Design review of the part built by this model. Coordinates are the model's own, in mm. A direction names the side the tool comes from. Coordinates: 2 decimals unless noted, no trailing zeros. Loops run counter-clockwise (first coordinate to the right, second up) from the corner with the lowest first, then second, coordinate; pieces in that order, holes last. Notation, with made-up numbers: (61, 42) -> (85, 42) arc R22 cw to (85, 77) -> close; hole circle Ø5 at (0.5, 54.5). An arc over 180 degrees is marked (long way). One line per item, written item: value. Start each with the question number.
1. Draft analysis for pull direction Z (two halves, no side actions). For faces 3 (the flat face through (-124.73, 0.021, -125.484)), 4 (the flat face through (-2, -1.511, -100)), 5 (the cylindrical face through (40.408, 0.021, -94.225)), 6 (the flat face through (-111.47, 0.02, -57.59)), state which applies: pulls with the +Z half, pulls with the -Z half, needs draft (parallel to the pull), parting line crosses it, or undercut.
2. Add section B-B on z = -55. Write out the cut boundary in (x, y), plus the area to 3 significant figures.
3. Machinability: for faces 1 (the flat face through (-64.801, 0.021, -20.804)), 2 (the flat face through (125.484, 0.021, -124.73)), which of the approach directions +Z, -Z, +X, -X, +Y, -Y give a long, thin tool a straight path to every point of the face, cutting with its end or side? Answer none if there is none.
4. For probe 1 along X at (y, z) = (0, -23); probe 2 along X at (y, z) = (-0.1, -66.5); probe 3 along Z at (x, y) = (71, -0.55), list the stretches that pass through material, from the lowest coordinate up.
5. Add section A-A on z = -81. Write out the cut boundary in (x, y).
6. Insertion check: pin 1 (1.5 mm diameter, centred on y = 0, z = -129, fed in from +X); pin 2 (3 mm diameter, centred on x = 24.46, z = -65.43, fed in from -Y); pin 3 (1 mm diameter, centred on x = 21, y = 0, fed in from +Z); pin 4 (1 mm diameter, centred on y = 1, z = -63, fed in from +X). Each pin has a flat end and moves straight along its axis. Give the tip position at first contact, or say it passes through.
7. Add section D-D on z = -142.5. Write out the cut boundary in (x, y) (3 decimals), plus the area to 3 significant figures.
8. Add section C-C on y = 1. Give the number of separate pieces and of enclosed holes in the cut face, plus the area to 3 significant figures.
```python
from build123d import *

# Parameters (mm, degrees)
BOSS_EXTRUDE1_DEPTH = 1.5113
SKETCH4_R           = 2.5527
CUT_EXTRUDE1_DEPTH  = 4.0226
CUT_EXTRUDE4_DEPTH  = 4.0226
SKETCH7_R           = 2.5527
CUT_EXTRUDE2_DEPTH  = 4.0226
SKETCH8_R           = 25.4
CUT_EXTRUDE3_DEPTH  = 4.0226


with BuildPart() as part:
    # Sketch3 → Boss-Extrude1 (new body, symmetric)
    with BuildSketch(Plane(origin=(0, 0, 0), x_dir=(1, 0, 0), z_dir=(0, 1, 0))):
        with BuildLine():
            Line((64.255461557, 10.37392483), (152.047852166, 98.16631544))
            Line((152.047852166, 98.16631544), (98.16631544, 152.047852166))
            Line((98.16631544, 152.047852166), (53.975, 152.047852166))
            Line((53.975, 152.047852166), (53.975, 120.65))
            Line((53.975, 120.65), (-53.975, 120.65))
            Line((-53.975, 120.65), (-53.975, 152.047852166))
            Line((-53.975, 152.047852166), (-98.16631544, 152.047852166))
            Line((-98.16631544, 152.047852166), (-152.047852166, 98.16631544))
            Line((-152.047852166, 98.16631544), (-64.255461557, 10.37392483))
            ThreePointArc((-64.255461557, 10.37392483), (0, 65.0875), (64.255461557, 10.37392483))
        make_face()
    extrude(amount=BOSS_EXTRUDE1_DEPTH, both=True)

    # Sketch4 → Cut-Extrude1 (cut, through all)
    with BuildSketch(Plane(origin=(0, 1.5113, 0), x_dir=(1, 0, 0), z_dir=(0, 1, 0))):
        with Locations((24.461985581, 65.426552419)):
            Circle(SKETCH4_R)
        with Locations((60.491874454, 34.925)):
            Circle(SKETCH4_R)
        with Locations((-60.491874454, 34.925)):
            Circle(SKETCH4_R)
        with Locations((-24.461985581, 65.426552419)):
            Circle(SKETCH4_R)
    extrude(amount=-CUT_EXTRUDE1_DEPTH, mode=Mode.SUBTRACT)

    # Sketch6 → Cut-Extrude4 (cut, through all)
    with BuildSketch(Plane(origin=(0, 1.5113, 0), x_dir=(1, 0, 0), z_dir=(0, 1, 0))):
        Polygon((69.743195158, 15.861658432), (60.762939037, 24.841914553), (59.718206073, 25.886647517), (64.255461557, 10.37392483), align=None)
    cut_extrude4 = extrude(amount=-CUT_EXTRUDE4_DEPTH, mode=Mode.SUBTRACT)

    # Sketch7 → Cut-Extrude2 (cut, through all)
    with BuildSketch(Plane(origin=(0, 1.5113, 0), x_dir=(1, 0, 0), z_dir=(0, 1, 0))):
        with Locations((70.865727173, 23.719382538)):
            Circle(SKETCH7_R)
        with Locations((79.845983295, 32.699638659)):
            Circle(SKETCH7_R)
    cut_extrude2 = extrude(amount=-CUT_EXTRUDE2_DEPTH, mode=Mode.SUBTRACT)

    # Mirror1: Cut-Extrude4, Cut-Extrude2 across plane
    add(cut_extrude4.mirror(Plane(origin=(0, 0, 0), x_dir=(0, 0, 1), z_dir=(1, 0, 0))), mode=Mode.SUBTRACT)
    add(cut_extrude2.mirror(Plane(origin=(0, 0, 0), x_dir=(0, 0, 1), z_dir=(1, 0, 0))), mode=Mode.SUBTRACT)

    # Sketch8 → Cut-Extrude3 (cut, through all)
    with BuildSketch(Plane(origin=(0, 1.5113, 0), x_dir=(1, 0, 0), z_dir=(0, 1, 0))):
        with Locations((59.128754095, 77.058092601)):
            Circle(SKETCH8_R)
    extrude(amount=-CUT_EXTRUDE3_DEPTH, mode=Mode.SUBTRACT)


solid = part.part
```
Worked answers:
1. face 3: pulls with the -Z half
1. face 4: needs draft
1. face 5: undercut
1. face 6: pulls with the +Z half
2. outline: (-108.88, -1.51) -> (-34.8, -1.51) -> (-34.8, 1.51) -> (-108.88, 1.51) -> close; (34.8, -1.51) -> (46.54, -1.51) -> (46.54, 1.51) -> (34.8, 1.51) -> close; (71.72, -1.51) -> (108.88, -1.51) -> (108.88, 1.51) -> (71.72, 1.51) -> close
2. area: 372 mm²
3. face 1: +Z, +Y, -Y
3. face 2: -Z, +X, +Y, -Y
4. probe 1: x = -76.88 to -73.31, -68.42 to -62.6, 62.6 to 68.42, 73.31 to 76.88
4. probe 2: x = -120.38 to -26.78, -22.15 to 22.15, 26.78 to 36.03, 82.23 to 120.38
4. probe 3: z = -152.05 to -99.51, -54.6 to -26.27, -21.17 to -17.12
5. outline: (-134.88, -1.51) -> (34.04, -1.51) -> (34.04, 1.51) -> (-134.88, 1.51) -> close; (84.22, -1.51) -> (134.88, -1.51) -> (134.88, 1.51) -> (84.22, 1.51) -> close
6. pin 1: stops at x = 121.96
6. pin 2: passes through
6. pin 3: stops at z = -61.43
6. pin 4: stops at x = 117.38
7. outline: (-107.714, -1.511) -> (-53.975, -1.511) -> (-53.975, 1.511) -> (-107.714, 1.511) -> close; (53.975, -1.511) -> (107.714, -1.511) -> (107.714, 1.511) -> (53.975, 1.511) -> close
7. area: 325 mm²
8. separate pieces: 1
8. enclosed holes: 9
8. area: 21,500 mm²
